from build123d import *

# Parameters (mm, degrees)
BOSS_EXTRUDE2_DEPTH     = 280
BOSS_EXTRUDE3_START     = 150
SKETCH5_R               = 140
BOSS_EXTRUDE3_DEPTH     = 30
BOSS_EXTRUDE4_START     = -150
SKETCH5_2_R             = 140
BOSS_EXTRUDE4_DEPTH     = 30
SKETCH6_R               = 25
CUT_EXTRUDE1_DEPTH      = 181
CUT_EXTRUDE1_DEPTH_BACK = 181
SKETCH7_R               = 37.5
BOSS_EXTRUDE5_DEPTH     = 325


with BuildPart() as part:
    # Sketch4 → Boss-Extrude2 (new body)
    with BuildSketch(Plane.XY):
        with BuildLine():
            Line((-130, 0), (130, 0))
            ThreePointArc((130, 0), (165.355339059, 14.644660941), (180, 50))
            Line((180, 50), (180, 380))
            Line((180, 380), (150, 380))
            Line((150, 380), (150, 50))
            ThreePointArc((150, 50), (144.142135624, 35.857864376), (130, 30))
            Line((130, 30), (-130, 30))
            ThreePointArc((-130, 30), (-144.142135624, 35.857864376), (-150, 50))
            Line((-150, 50), (-150, 380))
            Line((-150, 380), (-180, 380))
            Line((-180, 380), (-180, 50))
            ThreePointArc((-180, 50), (-165.355339059, 14.644660941), (-130, 0))
        make_face()
    extrude(amount=-BOSS_EXTRUDE2_DEPTH)

    # Sketch5 → Boss-Extrude3 (add)
    with BuildSketch(Plane(origin=(0, 0, 0), x_dir=(0, 0, -1), z_dir=(1, 0, 0)).offset(BOSS_EXTRUDE3_START)):
        with Locations((140, 380)):
            Circle(SKETCH5_R)
    extrude(amount=BOSS_EXTRUDE3_DEPTH)

    # Sketch5<2> → Boss-Extrude4 (add)
    with BuildSketch(Plane(origin=(0, 0, 0), x_dir=(0, 0, -1), z_dir=(1, 0, 0)).offset(BOSS_EXTRUDE4_START)):
        with Locations((140, 380)):
            Circle(SKETCH5_2_R)
    extrude(amount=-BOSS_EXTRUDE4_DEPTH)

    # Sketch6 → Cut-Extrude1 (cut, two sides)
    with BuildSketch(Plane(origin=(0, 0, 0), x_dir=(0, 0, -1), z_dir=(1, 0, 0))) as cut_extrude1_sk:
        with Locations((140, 380)):
            Circle(SKETCH6_R)
    extrude(amount=CUT_EXTRUDE1_DEPTH, mode=Mode.SUBTRACT)
    extrude(cut_extrude1_sk.sketch, amount=-CUT_EXTRUDE1_DEPTH_BACK, mode=Mode.SUBTRACT)

    # Sketch7 → Boss-Extrude5 (add)
    with BuildSketch(Plane(origin=(0, 0, 0), x_dir=(1, 0, 0), z_dir=(0, 1, 0))):
        with Locations((0, 140)):
            Circle(SKETCH7_R)
    extrude(amount=-BOSS_EXTRUDE5_DEPTH)


solid = part.part
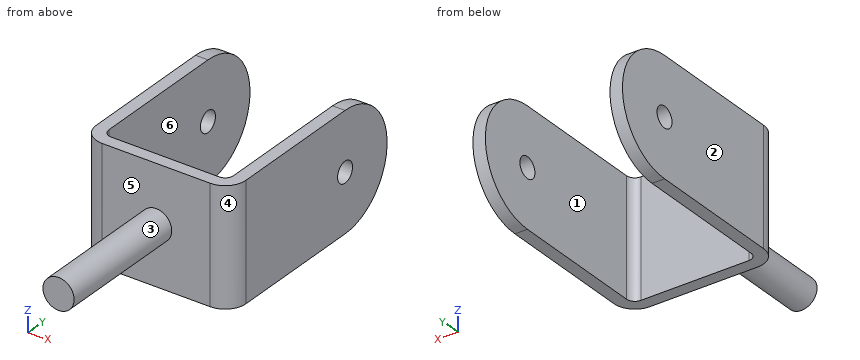
Geometry: final body of the model. Coordinates: model frame, mm. Face numbers are marked on the shaded views. A direction names the side the tool comes from. Round coordinates to 2 decimals unless told otherwise and drop trailing zeros. Loops run counter-clockwise (first coordinate to the right, second up) from the corner with the lowest first, then second, coordinate; pieces in that order, holes last.
Q1. Section B-B on y = 218.5. Return loops of the section in (x, z), plus the area to 3 significant figures.
Q2. Section A-A on z = -140. Return loops of the section in (x, y), plus the area to 3 significant figures.
Q3. Material intervals for L1, parallel to X at y = 131, z = -47; L2, parallel to Y at x = -21, z = -225.5; L3, parallel to Y at x = -166.5, z = -140, sorted ascending.
Q4. Section D-D on z = -236. Return loops of the section in (x, y).
Q5. Pin query (flat end, axial travel): P1, Ø1, axis at x = -139, z = -166, coming from the -Y side; P2, Ø2, axis at y = -141.5, z = -153.5, coming from the -X side. Return the tip coordinate at first contact, or that it passes through.
Q6. Pull-direction query (X, two-part tool) for the marked faces 1, 2 and 3; classes: released by +X, released by -X, zero draft, split by the parting line, or undercut.
Q7. Section C-C on x = 0. Return loops of the section in (y, z).
Q8. Access query for the marked faces 4, 5 and 6. Directions: +Z, -Z, +X, -X, +Y, -Y. A direction counts if a zero-diameter tool reaches every point of the face in a straight line with its end or side. Return the directions, or none.
Evaluation:
1. outline: (-180, -280) - (-150, -280) - (-150, 0) - (-180, 0) - close; (150, -280) - (180, -280) - (180, 0) - (150, 0) - close
1. area: 16,800 mm2
2. outline: (-180, 50) arc R50 ccw to (-130, 0) - (-37.5, 0) - (-37.5, -325) - (37.5, -325) - (37.5, 0) - (130, 0) arc R50 ccw to (180, 50) - (180, 355) - (150, 355) - (150, 50) arc R20 cw to (130, 30) - (-130, 30) arc R20 cw to (-150, 50) - (-150, 355) - (-180, 355) - close; (-180, 405) - (-150, 405) - (-150, 520) - (-180, 520) - close; (150, 405) - (180, 405) - (180, 520) - (150, 520) - close
2. area: 60,700 mm2
3. L1: x = -180 to -150, 150 to 180
3. L2: y = 0 to 30
3. L3: y = 15.83 to 355, 405 to 520
4. outline: (-180, 50) arc R50 ccw to (-130, 0) - (130, 0) arc R50 ccw to (180, 50) - (180, 481.9) - (150, 481.9) - (150, 50) arc R20 cw to (130, 30) - (-130, 30) arc R20 cw to (-150, 50) - (-150, 481.9) - (-180, 481.9) - close
5. P1: stops at y = 0.73
5. P2: stops at x = -35.36
6. face 1: undercut
6. face 2: released by -X
6. face 3: split by the parting line
7. outline: (-325, -177.5) - (0, -177.5) - (0, -280) - (30, -280) - (30, 0) - (0, 0) - (0, -102.5) - (-325, -102.5) - close
8. face 4: +Z, -Z, +X, -Y
8. face 5: -Y
8. face 6: +Z, -Z, +Y
